Here's how the part is built. I have some questions about the finished solid (model axes, mm). A direction names the side the tool comes from. Coordinates: 2 decimals unless noted, no trailing zeros. Order: outer loops, then holes, each group sorted by start corner. A loop starts at its lowest first (then second) coordinate and runs counter-clockwise, first axis right, second up. Notation, with made-up numbers: (66, 25.5) - (79, 25.5) arc R20 cw to (79, 56.5) - close; hole circle Ø7 at (47.25, 55). An arc over 180 degrees is marked (long way). Answer in a Markdown table with one row per item. Add a question column.
Item 1: I want a section at B-B (x = -1). Please give me the cut outline in (y, z).
Item 2: On a 3-axis mill with a long thin cutter (end or side, diameter ignored), from which of +Z, -Z, +X, -X, +Y, -Y can I reach the whole of each face in a straight line? I mean faces 1 (the flat face through (10, 40, 40)), 2 (the cylindrical face through (64.65, 10.623, 35.595)), 3 (the flat face through (-13, 20, 40)). Say none if no direction works.
Item 3: I want a section at C-C (y = -5.5). Please give me the cut outline in (x, z), plus the area to 3 significant figures.
Item 4: I want a section at D-D (y = 27). Please give me the cut outline in (x, z), plus the area to 3 significant figures.
Item 5: If I drill on line 1 along Y through (x, z) = (-14, 33); line 2 along X through (y, z) = (23, 37); line 3 along Y through (x, z) = (10.5, 51.5), over which ranges is the centre line in solid material (lowest first)? Write a range as from..to.
Item 6: I want a section at A-A (z = 55.5). Please give me the cut outline in (x, y).
Item 7: Will this pin go through, and if not, where does the flat tip stop? pin 1 Ø4 at (y, z) = (11, 44.5) entering from -X.
Item 8: Thinking about a two-plate mould opening in Y: for faces 4 (the flat face through (40, -9, 49)), 5 (the flat face through (-12, -20, 40)), 6 (the cylindrical face through (15, 0, 40)), 7 (the flat face through (10, -40, 40)), which applies, +Y half, -Y half, draft (parallel to the pull), parting line (faces both ways), or undercut?
```python
from build123d import *

# Parameters (mm, degrees)
CROQUIS1_W              = 80
CROQUIS1_H              = 80
SALIENTE_EXTRUIR1_DEPTH = 80
CROQUIS3_R              = 11.5
SALIENTE_EXTRUIR2_DEPTH = 50
CORTAR_EXTRUIR1_START   = 28.499999898
CORTAR_EXTRUIR1_DEPTH   = 23.000000204
CORTAR_EXTRUIR2_DEPTH   = 80
CORTAR_EXTRUIR3_START   = 40
CROQUIS7_W              = 20
CROQUIS7_H              = 80
CORTAR_EXTRUIR3_DEPTH   = 60


# Read off the part's stored shape, not the designer's step: Cortar-Extruir1
with BuildPart() as part:
    # Croquis1 → Saliente-Extruir1 (new body)
    with BuildSketch(Plane.XY):
        Rectangle(CROQUIS1_W, CROQUIS1_H)
    extrude(amount=SALIENTE_EXTRUIR1_DEPTH)

    # Croquis3 → Saliente-Extruir2 (add)
    with BuildSketch(Plane(origin=(40, 0, 0), x_dir=(0, 0, -1), z_dir=(1, 0, 0))):
        with Locations(Location((-40, 0, 0), (0, 0, 90))):
            Circle(CROQUIS3_R)
    extrude(amount=SALIENTE_EXTRUIR2_DEPTH)

    # Cortar-Extruir1 outline → Cortar-Extruir1 (cut)
    with BuildSketch(Plane.XY.offset(CORTAR_EXTRUIR1_START)):
        with BuildLine():
            add(Edge.make_bspline(
                [(57, 0), (57, 0.79647294), (57.328173799, 1.571048026), (58.430085354, 2.672492311), (59.211671862, 2.999496362), (60.78449026, 3.00050241), (61.565740512, 2.676816215), (62.676579515, 1.566145107), (62.999665754, 0.786423133), (63.000333703, -0.783870942), (62.675691102, -1.566206232), (61.569794846, -2.673587285), (60.79292663, -2.999619771), (59.20995314, -3.000379538), (58.430916235, -2.672841833), (57.329196069, -1.57255006), (57, -0.79647294), (57, 0)],
                knots=[0, 0, 0, 0, 0.125, 0.125, 0.25, 0.25, 0.375, 0.375, 0.5, 0.5, 0.625, 0.625, 0.75, 0.75, 0.875, 0.875, 1, 1, 1, 1], degree=3))
        make_face()
    extrude(amount=CORTAR_EXTRUIR1_DEPTH, mode=Mode.SUBTRACT)

    # Croquis5 → Cortar-Extruir2 (cut)
    with BuildSketch(Plane.XY.offset(80)):
        with BuildLine():
            Line((-20, 40), (-20, 20))
            Line((-20, 20), (-5, 20))
            ThreePointArc((-5, 20), (15, 0), (-5, -20))
            Line((-5, -20), (-20, -20))
            Line((-20, -20), (-20, -40))
            Line((-20, -40), (-40, -40))
            Line((-40, -40), (-40, 40))
            Line((-40, 40), (-20, 40))
        make_face()
    extrude(amount=-CORTAR_EXTRUIR2_DEPTH, mode=Mode.SUBTRACT)

    # Croquis7 → Cortar-Extruir3 (cut)
    with BuildSketch(Plane(origin=(0, 0, 0), x_dir=(0, 0, -1), z_dir=(1, 0, 0)).offset(CORTAR_EXTRUIR3_START)):
        with Locations((-70, 0)):
            Rectangle(CROQUIS7_W, CROQUIS7_H)
        with Locations((-10, 0)):
            Rectangle(CROQUIS7_W, CROQUIS7_H)
    extrude(amount=-CORTAR_EXTRUIR3_DEPTH, mode=Mode.SUBTRACT)


solid = part.part
```
Values follow:
| question | item | result |
|---|---|---|
| 1 | outline | (-40, 20) - (-19.6, 20) - (-19.6, 60) - (-40, 60) - close; (19.6, 20) - (40, 20) - (40, 60) - (19.6, 60) - close |
| 2 | face 1 | +Z, -Z, +X, -X, +Y |
| 2 | face 2 | +X |
| 2 | face 3 | +Z, -Z, -X |
| 3 | outline | (14.23, 20) - (40, 20) - (40, 29.9) - (90, 29.9) - (90, 50.1) - (40, 50.1) - (40, 60) - (14.23, 60) - close |
| 3 | area | 2,040 mm^2 |
| 4 | outline | (-20, 20) - (40, 20) - (40, 60) - (-20, 60) - close |
| 4 | area | 2,400 mm^2 |
| 5 | line 1 | y = -40..-20, 20..40 |
| 5 | line 2 | x = -20..40 |
| 5 | line 3 | y = -40..-12.64, 12.64..40 |
| 6 | outline | (-20, -40) - (40, -40) - (40, 40) - (-20, 40) - (-20, 20) - (-5, 20) arc R20 cw to (-5, -20) - (-20, -20) - close |
| 7 | pin 1 | stops at x = 10.2 |
| 8 | face 4 | draft |
| 8 | face 5 | undercut |
| 8 | face 6 | undercut |
| 8 | face 7 | -Y half |
